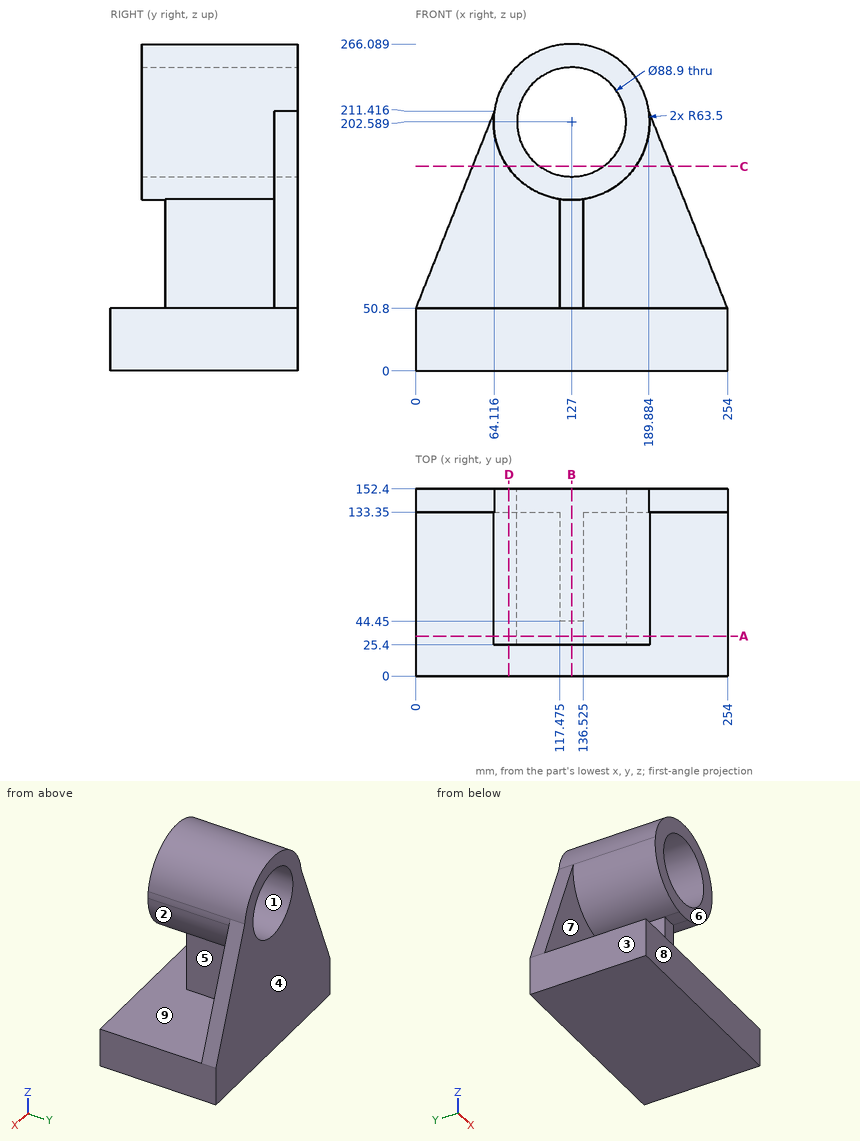
Check sheet for the drawn part. Datum: minimum x, y, z corner. Units: mm. A direction names the side the tool comes from. Round coordinates to 2 decimals unless told otherwise and drop trailing zeros. Order: outer loops, then holes, each group sorted by start corner. A loop starts at its lowest first (then second) coordinate and runs counter-clockwise, first axis right, second up.
1) Scan lines: line 1 (Z direction, x = 151.5, y = 64.5) (1 decimal); line 2 (Y direction, x = 72, z = 193); line 3 (X direction, y = 84, z = 60.5) (1 decimal). Record each from-to range of solid material in increasing order.
2) Section check A-A (y = 32.5). Give the number of separate pieces and of enclosed holes in the cut face, and give its area (3 significant figures).
3) Section check C-C (z = 166.5). Record the boundary of the cut face in (x, y).
4) Mould release check, pull along X, two halves, no side actions. Record for the marked faces 1, 2, 3 and 4: +X half, -X half, draft (parallel to the pull), parting line (faces both ways), or undercut.
5) Go/stop test with flat-tipped pins: pin 1 Ø5 at (x, y) = (159, 122.5) entering from +Z; pin 2 Ø3 at (y, z) = (45.5, 53) entering from +X (3 decimals); pin 3 Ø1.5 at (y, z) = (79.5, 189) entering from -X. Record where each tip stops, or that it passes through.
6) Tool access check on the marked faces 5, 6, 7, 8 and 9. Record the directions out of +Z, -Z, +X, -X, +Y, -Y that give a thin tool (end or side, any length) a straight path to the whole face; none if there is none.
7) Section check B-B (x = 127). Record the boundary of the cut face in (y, z), and give its area (3 significant figures).
8) Section check D-D (x = 76). Record the boundary of the cut face in (y, z), and give its area (3 significant figures).
Result:
1. line 1: z = 0 to 50.8, 144 to 165.5, 239.7 to 261.2
1. line 2: y = 25.4 to 152.4
1. line 3: x = 117.5 to 136.5
2. separate pieces: 2
2. enclosed holes: 1
2. area: 19,400 mm2
3. outline: (46.19, 133.35) - (74.75, 133.35) - (74.75, 25.4) - (101.05, 25.4) - (101.05, 152.4) - (46.19, 152.4) - close; (152.95, 25.4) - (179.25, 25.4) - (179.25, 133.35) - (207.81, 133.35) - (207.81, 152.4) - (152.95, 152.4) - close
4. face 1: undercut
4. face 2: +X half
4. face 3: -X half
4. face 4: draft
5. pin 1: stops at z = 258.82
5. pin 2: stops at x = 136.525
5. pin 3: stops at x = 64.81
6. face 5: +X, -Y
6. face 6: +Z, +X, -X, -Y
6. face 7: -X, -Y
6. face 8: +Z, -Z, +X, -X, -Y
6. face 9: -Y
7. outline: (0, 0) - (152.4, 0) - (152.4, 158.14) - (25.4, 158.14) - (25.4, 139.09) - (44.45, 139.09) - (44.45, 50.8) - (0, 50.8) - close; (25.4, 247.04) - (152.4, 247.04) - (152.4, 266.09) - (25.4, 266.09) - close
7. area: 22,100 mm2
8. outline: (0, 0) - (152.4, 0) - (152.4, 240.42) - (25.4, 240.42) - (25.4, 164.76) - (133.35, 164.76) - (133.35, 50.8) - (0, 50.8) - close
8. area: 19,500 mm2
